CAD build for the part. Positions are in the model's coordinates, mm. A direction names the side the tool comes from. Round coordinates to 2 decimals unless told otherwise and drop trailing zeros. Write each loop counter-clockwise with the first axis right and the second up, starting at its lowest first coordinate (ties: lowest second). Pieces come first, ordered by that corner, then holes. Notation, with made-up numbers: (25, 50) - (44, 50) arc R11 ccw to (44, 70) - close; hole circle Ø11 at (77, 63). An arc over 180 degrees is marked (long way). Answer in a Markdown table with one row per item.
```python
from build123d import *

# Parameters (mm, degrees)
F0_W     = 100
F0_H     = 100
F1_DEPTH = 50
F2_W     = 8.5
F2_H     = 8.5
F3_DEPTH = 56.75


with BuildPart() as f1:
    # F0 (on Top) → F1 (new body, symmetric)
    with BuildSketch(Plane.XY):
        Rectangle(F0_W, F0_H)
    extrude(amount=F1_DEPTH, both=True)

    # F2 (on Top) → F3 (join, symmetric)
    with BuildSketch(Plane.XY):
        with Locations((-45.75, 45.75)):
            Rectangle(F2_W, F2_H)
        with Locations((45.75, 45.75)):
            Rectangle(F2_W, F2_H)
        with Locations((45.75, -45.75)):
            Rectangle(F2_W, F2_H)
        with Locations((-45.75, -45.75)):
            Rectangle(F2_W, F2_H)
    extrude(amount=F3_DEPTH, both=True)


solid = f1.part
```
Q1. Saw through at B-B on y = -29. List the corners of the cut face in (x, z), then the cut area to 3 significant figures.
Computed:
| item | result |
|---|---|
| outline | (-50, -50) - (50, -50) - (50, 50) - (-50, 50) - close |
| area | 10,000 mm2 |
Q2. Drill centre line: line 1 (Z direction, x = -25, y = -46). Where is it in solid material? Low to high.
Computed:
| item | result |
|---|---|
| line 1 | z = -50 to 50 |
Q3. Saw through at A-A on x = 44. List the corners of the cut face in (y, z), then the cut area to 3 significant figures.
Computed:
| item | result |
|---|---|
| outline | (-50, -56.75) - (-41.5, -56.75) - (-41.5, -50) - (41.5, -50) - (41.5, -56.75) - (50, -56.75) - (50, 56.75) - (41.5, 56.75) - (41.5, 50) - (-41.5, 50) - (-41.5, 56.75) - (-50, 56.75) - close |
| area | 10,200 mm2 |
Q4. Flat gauge pins, fed straight in: pin 1 (10 mm diameter, centred on x = 23, y = 37, fed in from -Z); pin 2 (6 mm diameter, centred on x = 16.5, y = -13, fed in from +Z). Where does each tip first touch, or does it go through?
Computed:
| item | result |
|---|---|
| pin 1 | stops at z = -50 |
| pin 2 | stops at z = 50 |
Q5. Pull direction Y, two halves, no side cores. Call faces 5 (the flat face through (-46, -46, -56.75)), 6 (the flat face through (46, -41.5, -53)), 7 (the flat face through (-1, 50, 1)): released by +Y, released by -Y, zero draft, split by the parting line, or undercut.
Computed:
| item | result |
|---|---|
| face 5 | zero draft |
| face 6 | undercut |
| face 7 | released by +Y |
Q6. 3-axis set-ups, long thin cutter, end or side, ignore diameter. For faces 1 (the flat face through (41.5, -46, 53)), 2 (the flat face through (-46, -41.5, -53)), 3 (the flat face through (41.5, -46, -53)), 4 (the flat face through (46, -41.5, 53)): which of +Z, -Z, +X, -X, +Y, -Y reach the whole face in a straight line?
Computed:
| item | result |
|---|---|
| face 1 | +Z, +Y, -Y |
| face 2 | -Z, +X, -X |
| face 3 | -Z, +Y, -Y |
| face 4 | +Z, +X, -X |
